Design review of the part shown in the three views and the two pictorial views. Dimensions are in mm from the part's minimum x, y and z. A direction names the side the tool comes from. Give positions to 0.01 mm unless a question says otherwise; leave off trailing zeros. Loops run counter-clockwise (first coordinate to the right, second up) from the corner with the lowest first, then second, coordinate; pieces in that order, holes last. Notation, with made-up numbers: M 67.5,-14 L 79.5,-14 A31 cw 79.5,12 Z; hole C 40.5,19 d8. An arc over 180 degrees is marked long. Return JSON: item names as keys, results as strings. Group by question number.
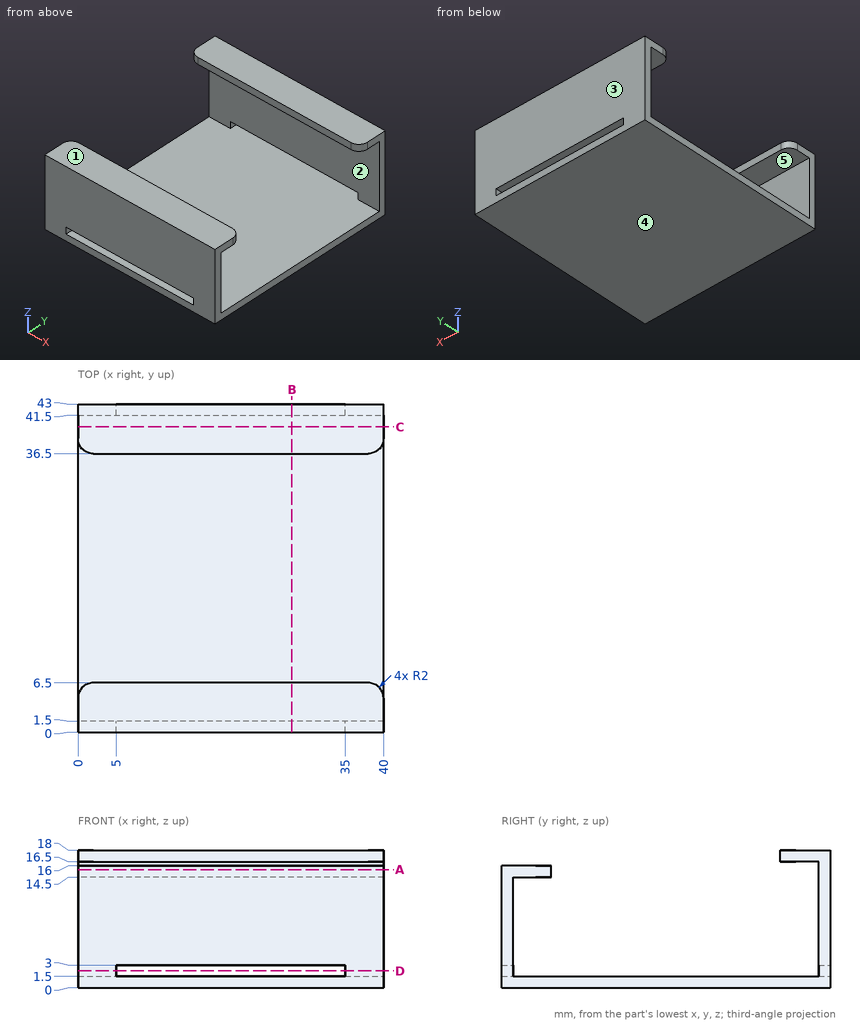
(1) For pin 1 (10 mm diameter, centred on x = 19.5, y = 11, fed in from +Z); pin 2 (12 mm diameter, centred on x = 25.5, y = 16.5, fed in from +Z), all flat-tipped, find the tip position at first contact; note any pin that passes through.
(2) For probe 1 along Y at (x, z) = (27, 3.5); probe 2 along Y at (x, z) = (33.5, 15.75); probe 3 along Z at (x, y) = (10.5, 29), list the stretches that pass through material, from the lowest coordinate up.
(3) Add section B-B (x = 28). Write out the cut boundary in (y, z), and give its area (4 significant figures).
(4) Add section C-C (y = 40). Write out the cut boundary in (x, z), and give its area (3 significant figures).
(5) Mouldability with a two-part tool opening along Y and no side actions: class the marked faces 1, 2 and 3 as released by +Y, released by -Y, zero draft, split by the parting line, or undercut.
(6) For the marked faces 4 and 5, list the 3-axis set-ups (+Z, -Z, +X, -X, +Y, -Y) from which the entire face can be reached by the end or side of a thin tool; tool diameter is ignored.
(7) Add section D-D (z = 2.25). Write out the cut boundary in (x, y), and give its area (3 significant figures).
(8) Add section A-A (z = 15.5). Write out the cut boundary in (x, y), and give its area (3 significant figures).
Verdict:
{
 "1": {"pin 1": "stops at z = 16", "pin 2": "stops at z = 1.5"},
 "2": {"probe 1": "y = 0 to 1.5, 41.5 to 43", "probe 2": "y = 0 to 6.5, 41.5 to 43", "probe 3": "z = 0 to 1.5"},
 "3": {"outline": "M 0,0 L 43,0 L 43,1.5 L 0,1.5 Z; M 0,3 L 1.5,3 L 1.5,14.5 L 6.5,14.5 L 6.5,16 L 0,16 Z; M 36.5,16.5 L 41.5,16.5 L 41.5,3 L 43,3 L 43,18 L 36.5,18 Z", "area": "121.5 mm²"},
 "4": {"outline": "M 0,0 L 40,0 L 40,1.5 L 0,1.5 Z; M 0,16.5 L 40,16.5 L 40,18 L 0,18 Z", "area": "120 mm²"},
 "5": {"face 1": "zero draft", "face 2": "undercut", "face 3": "released by +Y"},
 "6": {"face 4": "-Z, +X, -X, +Y, -Y", "face 5": "+X, -X"},
 "7": {"outline": "M 0,0 L 5,0 L 5,1.5 L 0,1.5 Z; M 0,41.5 L 5,41.5 L 5,43 L 0,43 Z; M 35,0 L 40,0 L 40,1.5 L 35,1.5 Z; M 35,41.5 L 40,41.5 L 40,43 L 35,43 Z", "area": "30.0 mm²"},
 "8": {"outline": "M 0,0 L 40,0 L 40,4.5 A2 ccw 38,6.5 L 2,6.5 A2 ccw 0,4.5 Z; M 0,41.5 L 40,41.5 L 40,43 L 0,43 Z", "area": "318 mm²"}
}
